Can you work these out from the model? Positions are in its coordinate system, mm. Give positions to 0.01 mm unless a question says otherwise; leave off trailing zeros. Order: outer loops, then holes, each group sorted by start corner. A loop starts at its lowest first (then second) coordinate and runs counter-clockwise, first axis right, second up. Notation, with made-up numbers: (73.25, 10) -> (83.25, 10) arc R10 cw to (83.25, 21) -> close; hole circle Ø1 at (78.5, 16). An arc over 180 degrees is marked (long way). Answer as CSV lines item,"result".
```python
from build123d import *

# Parameters (mm, degrees)
SKETCH1_W           = 30
SKETCH1_H           = 50
SKETCH1_R           = 4
BOSS_EXTRUDE1_DEPTH = 6
FILLET1_R           = 0.5


with BuildPart() as part:
    # Sketch1 → Boss-Extrude1 (new body)
    with BuildSketch(Plane.XY):
        Rectangle(SKETCH1_W, SKETCH1_H)
        with Locations((-7.5, 0)):
            Circle(SKETCH1_R, mode=Mode.SUBTRACT)
        with Locations((7.5, 0)):
            Circle(SKETCH1_R, mode=Mode.SUBTRACT)
    extrude(amount=BOSS_EXTRUDE1_DEPTH)

    # Fillet1
    fillet1_edges = [part.edges().sort_by_distance(p)[0] for p in [
        (-15, 0, 6),
        (0, -25, 6),
        (15, 0, 6),
        (0, -25, 0),
        (-15, 0, 0),
        (0, 25, 0),
        (15, 0, 0),
        (15, -25, 3),
        (-15, -25, 3),
        (-15, 25, 3),
        (15, 25, 3),
        (0, 25, 6),
    ]]
    fillet(fillet1_edges, radius=FILLET1_R)


solid = part.part
```
Item 1: Imagine slicing it at B-B, the plane x = -7.5. Please give me the cut outline in (y, z), then the cut area to 3 significant figures.
Numbers:
outline,"(-25, 0.5) arc R0.5 ccw to (-24.5, 0) -> (-4, 0) -> (-4, 6) -> (-24.5, 6) arc R0.5 ccw to (-25, 5.5) -> close; (4, 0) -> (24.5, 0) arc R0.5 ccw to (25, 0.5) -> (25, 5.5) arc R0.5 ccw to (24.5, 6) -> (4, 6) -> close"
area,"252 mm²"
Item 2: For pin 1 (13 mm diameter, centred on x = -7.5, y = 0, fed in from -Z), with a flat end and sliding along its axis, tell me the tip position at first contact or that it passes through.
Numbers:
pin 1,"stops at z = 0"
Item 3: Please list where these lines run through material, in increasing order: line 1 along Y through (x, z) = (7.5, 2.4); line 2 along X through (y, z) = (-0.5, 1.15); line 3 along Y through (x, z) = (-10.5, 3.8).
Numbers:
line 1,"y = -25 to -4, 4 to 25"
line 2,"x = -15 to -11.47, -3.53 to 3.53, 11.47 to 15"
line 3,"y = -25 to -2.65, 2.65 to 25"
Item 4: We'd pull the mould along Y, two halves only. Please class faces 1 (the flat face through (-15, 0, 3)), 2 (the flat face through (0, 25, 3)), 3 (the cylindrical face through (4.3, -2.4, 3)): released by +Y, released by -Y, zero draft, split by the parting line, or undercut.
Numbers:
face 1,"zero draft"
face 2,"released by +Y"
face 3,"undercut"
Item 5: Imagine slicing it at A-A, the plane y = 0. Please give me the cut outline in (x, z), then the cut area to 3 significant figures.
Numbers:
outline,"(-15, 0.5) arc R0.5 ccw to (-14.5, 0) -> (-11.5, 0) -> (-11.5, 6) -> (-14.5, 6) arc R0.5 ccw to (-15, 5.5) -> close; (-3.5, 0) -> (3.5, 0) -> (3.5, 6) -> (-3.5, 6) -> close; (11.5, 0) -> (14.5, 0) arc R0.5 ccw to (15, 0.5) -> (15, 5.5) arc R0.5 ccw to (14.5, 6) -> (11.5, 6) -> close"
area,"83.8 mm²"
Item 6: Imagine slicing it at C-C, the plane z = 2.3. Please give me the cut outline in (x, y), then the cut area to 3 significant figures.
Numbers:
outline,"(-15, -24.5) arc R0.5 ccw to (-14.5, -25) -> (14.5, -25) arc R0.5 ccw to (15, -24.5) -> (15, 24.5) arc R0.5 ccw to (14.5, 25) -> (-14.5, 25) arc R0.5 ccw to (-15, 24.5) -> close; hole circle Ø8 at (-7.5, 0); hole circle Ø8 at (7.5, 0)"
area,"1,400 mm²"
